Autodesk Inventor part; units mm, degrees
ref_plane "YZ Plane" through (0, 0, 0) normal (1, 0, 0) x (0, 1, 0)
ref_plane "XZ Plane" through (0, 0, 0) normal (0, 1, 0) x (-1, 0, 0)
ref_plane "XY Plane" through (0, 0, 0) normal (0, 0, 1) x (1, 0, 0)
sketch "Sketch1" plane through (0, 0, 0) normal (0, 0, 1) x (1, 0, 0)
  circle A0 centre (0, 0) radius 30
  dimension "d0" = 60
extrude "Extrusion1" add sketch "Sketch1" along normal blind 3
sketch "Sketch2" plane through (0, 0, 0) normal (0, 0, -1) x (-1, 0, 0)
  circle A0 centre (0, 0) radius 10
  dimension "d3" = 20
extrude "Extrusion2" add sketch "Sketch2" along normal blind 4
sketch "Sketch3" plane through (0, 0, 3) normal (0, 0, 1) x (1, 0, 0)
  point P0 (0, 0)
  point P1 (0, 0)
hole "Hole1" at (0, 0, 3) direction (0, 0, -1) diameter 1 end through all
equation "\"d0\" = re_diametro"
equation "\"d1\" = re_grosor"
equation "\"d3\" = re_eje_diametro"
equation "\"d4\" = re_eje_grosor"
equation "\"d6\" = ri_ancla_diametro"
properties part number "Rueda Externa"
Design review of the part built by this model. Coordinates are the model's own, in mm. A direction names the side the tool comes from. Give positions to 0.01 mm unless a question says otherwise; leave off trailing zeros. Order: outer loops, then holes, each group sorted by start corner. A loop starts at its lowest first (then second) coordinate and runs counter-clockwise, first axis right, second up. Notation, with made-up numbers: (12, 16) -> (26, 16) arc R22 cw to (26, 39) -> close; hole circle Ø7 at (-6.5, -25.75). An arc over 180 degrees is marked (long way). Write item = value, one per line. Start each with the question number.
(1) To check wall thickness, follow line 1 along Y through (x, z) = (0, 1.5); line 2 along Y through (x, z) = (0, -2.5); line 3 along Z through (x, y) = (4, 26). State the ranges of each line that lie inside material, in increasing order.
(2) We need section D-D on x = 18. Write out the cut boundary in (y, z).
(3) For faces 1 (the face through (-2, 0, -4)), 2 (the face through (13, 0, 0)), list the 3-axis set-ups (+Z, -Z, +X, -X, +Y, -Y) from which the entire face can be reached by the end or side of a thin tool; tool diameter is ignored.
(4) We need section C-C on y = -24. Write out the cut boundary in (x, z).
(5) For pin 1 (2 mm diameter, centred on x = -16, z = -2, fed in from -Y); pin 2 (6 mm diameter, centred on x = -21.5, y = -19.5, fed in from -Z); pin 3 (1 mm diameter, centred on y = -1, z = 1.5, fed in from +X); pin 4 (2 mm diameter, centred on x = -21, z = 2, fed in from +Y), all flat-tipped, find the tip position at first contact; note any pin that passes through.
(6) We need section B-B on z = 2.25. Write out the cut boundary in (x, y), plus the area to 3 significant figures.
(7) We need section A-A on x = 3. Write out the cut boundary in (y, z).
Numbers:
q1.line_1 = -30 to -0.5, 0.5 to 30
q1.line_2 = -10 to -0.5, 0.5 to 10
q1.line_3 = 0 to 3
q2.outline = (-24, 0) -> (24, 0) -> (24, 3) -> (-24, 3) -> close
q3.face_1 = -Z, +X, -X, +Y, -Y
q3.face_2 = -Z
q4.outline = (-18, 0) -> (18, 0) -> (18, 3) -> (-18, 3) -> close
q5.pin_1 = through
q5.pin_2 = 0
q5.pin_3 = 30
q5.pin_4 = 22.36
q6.outline = circle Ø60 at (0, 0); hole circle Ø1 at (0, 0)
q6.area = 2,830 mm^2
q7.outline = (-29.85, 0) -> (-9.54, 0) -> (-9.54, -4) -> (9.54, -4) -> (9.54, 0) -> (29.85, 0) -> (29.85, 3) -> (-29.85, 3) -> close
